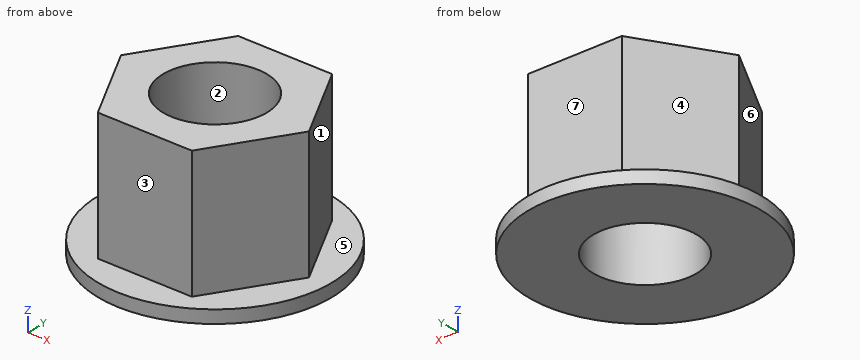
from build123d import *

# Parameters (mm, degrees)
SKETCH_R     = 18
PAD_DEPTH    = 2
PAD001_DEPTH = 20
SKETCH002_R  = 8
POCKET_DEPTH = 22


with BuildPart() as part:
    # Sketch → Pad (new body)
    with BuildSketch(Plane.XY):
        Circle(SKETCH_R)
    extrude(amount=PAD_DEPTH)

    # Sketch001 (on Face3 of Pad) → Pad001 (join)
    with BuildSketch(Plane.XY.offset(2)):
        Polygon((15, 0), (7.5, 12.990381), (-7.5, 12.990381), (-15, 0), (-7.5, -12.990381), (7.5, -12.990381), align=None)
    extrude(amount=PAD001_DEPTH)

    # Sketch002 (on Face10 of Pad001) → Pocket (cut)
    with BuildSketch(Plane.XY.offset(22)):
        Circle(SKETCH002_R)
    extrude(amount=-POCKET_DEPTH, mode=Mode.SUBTRACT)


solid = part.part
For this review, take the finished solid that the model builds, in its own axes (mm). Face numbers are marked on the shaded views. A direction names the side the tool comes from. Round coordinates to 2 decimals unless told otherwise and drop trailing zeros. Order: outer loops, then holes, each group sorted by start corner. A loop starts at its lowest first (then second) coordinate and runs counter-clockwise, first axis right, second up. Notation, with made-up numbers: M 52,41 L 59,41 A23 ccw 59,55 Z; hole C 51.25,-27 d5. An arc over 180 degrees is marked long. Use a Markdown table: item, result. Add a question column.
Item 1: Add section D-D, the plane x = -12.5. Give the boundary of the cut face in (y, z).
Item 2: Insertion check: pin 1 (5 mm diameter, centred on x = 14, y = 12, fed in from +Z); pin 2 (4.5 mm diameter, centred on x = 1, z = 11, fed in from +Y); pin 3 (1 mm diameter, centred on y = 11, z = 19.5, fed in from -X). Each pin has a flat end and moves straight along its axis. Give the tip position at first contact, or say it passes through.
Item 3: Add section C-C, the plane y = 2.5. Give the boundary of the cut face in (x, z), then the cut area to 3 significant figures.
Item 4: Tool access review of the marked faces 4, 5, 6 and 7: name each direction out of +Z, -Z, +X, -X, +Y, -Y from which nothing blocks a thin tool from reaching the whole face with its end or side.
Item 5: Add section B-B, the plane x = 0. Give the boundary of the cut face in (y, z).
Item 6: Mouldability with a two-part tool opening along X and no side actions: class the marked faces 1, 2 and 3 as released by +X, released by -X, zero draft, split by the parting line, or undercut.
Item 7: To check wall thickness, follow line 1 along Y through (x, z) = (0, 17); line 2 along Y through (x, z) = (4.5, 9.75); line 3 along X through (y, z) = (1.5, 3.5). State the ranges of each line that lie inside material, in increasing order.
Item 8: Add section A-A, the plane z = 7.5. Give the boundary of the cut face in (x, y).
Geometry results:
| question | item | result |
|---|---|---|
| 1 | outline | M -12.95,0 L 12.95,0 L 12.95,2 L 4.33,2 L 4.33,22 L -4.33,22 L -4.33,2 L -12.95,2 Z |
| 2 | pin 1 | stops at z = 2 |
| 2 | pin 2 | stops at y = 12.99 |
| 2 | pin 3 | stops at x = -8.94 |
| 3 | outline | M -17.83,0 L -7.6,0 L -7.6,22 L -13.56,22 L -13.56,2 L -17.83,2 Z; M 7.6,0 L 17.83,0 L 17.83,2 L 13.56,2 L 13.56,22 L 7.6,22 Z |
| 3 | area | 279 mm² |
| 4 | face 4 | +Z, -X, +Y |
| 4 | face 5 | +Z |
| 4 | face 6 | +Z, -X, -Y |
| 4 | face 7 | +Z, +X, -X, +Y |
| 5 | outline | M -18,0 L -8,0 L -8,22 L -12.99,22 L -12.99,2 L -18,2 Z; M 8,0 L 18,0 L 18,2 L 12.99,2 L 12.99,22 L 8,22 Z |
| 6 | face 1 | released by +X |
| 6 | face 2 | undercut |
| 6 | face 3 | zero draft |
| 7 | line 1 | y = -12.99 to -8, 8 to 12.99 |
| 7 | line 2 | y = -12.99 to -6.61, 6.61 to 12.99 |
| 7 | line 3 | x = -14.13 to -7.86, 7.86 to 14.13 |
| 8 | outline | M -15,0 L -7.5,-12.99 L 7.5,-12.99 L 15,0 L 7.5,12.99 L -7.5,12.99 Z; hole C 0,0 d16 |
